from build123d import *

# Parameters (mm, degrees)
SKETCH016_R     = 3
PAD007_DEPTH    = 4
SKETCH023_R     = 1.8
POCKET007_DEPTH = 6
CHAMFER001_SIZE = 0.3


with BuildPart() as part:
    # Sketch016 → Pad007 (new body)
    with BuildSketch(Plane.XY.offset(11)):
        Circle(SKETCH016_R)
    extrude(amount=PAD007_DEPTH)

    # Sketch023 (on Face3 of Pad007) → Pocket007 (cut)
    with BuildSketch(Plane.XY.offset(15)):
        Circle(SKETCH023_R)
    extrude(amount=-POCKET007_DEPTH, mode=Mode.SUBTRACT)

    # Chamfer001
    chamfer001_edges = [part.edges().sort_by_distance(p)[0] for p in [
        (-3, 0, 15),
    ]]
    chamfer(chamfer001_edges, length=CHAMFER001_SIZE)


with BuildPart() as part_1:
    # Body002 placement: moved
    add(part.part.moved(Location((0, 0, -1))))


solid = part_1.part
Verification items for the finished model (mm, model axes). Round coordinates to 2 decimals unless told otherwise and drop trailing zeros. Loops run counter-clockwise (first coordinate to the right, second up) from the corner with the lowest first, then second, coordinate; pieces in that order, holes last. Notation, with made-up numbers: (65.25, 26.25) - (111.25, 26.25) arc R26 cw to (111.25, 42.25) - close; hole circle Ø2 at (35, 15.5). An arc over 180 degrees is marked (long way). Write item = value, one per line.
Q1. Sectioned sample at C-C on z = 13.1. Record the boundary of the cut face in (x, y), plus the area to 3 significant figures.
Here are the results:
outline = circle Ø6 at (0, 0); hole circle Ø3.6 at (0, 0)
area = 18.1 mm^2
Q2. Depth check by flat-ended pin: pin 1 (2 mm diameter, centred on y = 1.5, z = 12, fed in from +X); pin 2 (2 mm diameter, centred on x = -1, z = 11.5, fed in from -Y); pin 3 (1.5 mm diameter, centred on y = 1.5, z = 11, fed in from -X). Enter the tip coordinate at first touch or a pass-through.
Here are the results:
pin_1 = 2.96
pin_2 = -3
pin_3 = -2.9
Q3. Sectioned sample at A-A on y = 0. Record the boundary of the cut face in (x, z).
Here are the results:
outline = (-3, 10) - (-1.8, 10) - (-1.8, 14) - (-2.7, 14) - (-3, 13.7) - close; (1.8, 10) - (3, 10) - (3, 13.7) - (2.7, 14) - (1.8, 14) - close
Q4. Material ranges on L1, parallel to Y at x = 0, z = 12.5; L2, parallel to X at y = -1.4, z = 10.4; L3, parallel to X at y = -1, z = 11.9, recorded low to high.
Here are the results:
L1 = -3 to -1.8, 1.8 to 3
L2 = -2.65 to -1.13, 1.13 to 2.65
L3 = -2.83 to -1.5, 1.5 to 2.83
